from build123d import *

# Parameters (mm, degrees)
F1_DEPTH = 1


with BuildPart() as f1:
    # F0 (on Front) → F1 (new body)
    with BuildSketch(Plane.XZ):
        with BuildLine():
            Line((29.8694758117, 20.3505297415), (-28.1305241883, 20.3505297415))
            ThreePointArc((-28.1305241883, 20.3505297415), (-29.5447377507, 19.7647433039), (-30.1305241883, 18.3505297415))
            Line((-30.1305241883, 18.3505297415), (-30.1305241883, 10.3505297415))
            Line((-30.1305241883, 10.3505297415), (-29.0812929486, 3.7248891079))
            ThreePointArc((-29.0812929486, 3.7248891079), (-25.1305241883, 0.3505297415), (-21.179755428, 3.7248891079))
            Line((-21.179755428, 3.7248891079), (-20.1305241883, 10.3505297415))
            ThreePointArc((-20.1305241883, 10.3505297415), (-18.6660580942, 13.8860636474), (-15.1305241883, 15.3505297415))
            Line((-15.1305241883, 15.3505297415), (-13.2839401439, 15.3505297415))
            Line((-13.2839401439, 15.3505297415), (-4.2025822867, 15.3505297415))
            ThreePointArc((-4.2025822867, 15.3505297415), (-0.6670483807, 13.8860636474), (0.7974177133, 10.3505297415))
            ThreePointArc((0.7974177133, 10.3505297415), (2.2618838074, 6.8149958356), (5.7974177133, 5.3505297415))
            ThreePointArc((5.7974177133, 5.3505297415), (9.3329516193, 6.8149958356), (10.7974177133, 10.3505297415))
            ThreePointArc((10.7974177133, 10.3505297415), (12.2618838074, 13.8860636474), (15.7974177133, 15.3505297415))
            Line((15.7974177133, 15.3505297415), (27.8694758117, 15.3505297415))
            Line((27.8694758117, 15.3505297415), (61.8694758117, 15.3505297415))
            Line((61.8694758117, 15.3505297415), (73.9415339101, 15.3505297415))
            ThreePointArc((73.9415339101, 15.3505297415), (77.477067816, 13.8860636474), (78.9415339101, 10.3505297415))
            ThreePointArc((78.9415339101, 10.3505297415), (80.4060000042, 6.8149958356), (83.9415339101, 5.3505297415))
            ThreePointArc((83.9415339101, 5.3505297415), (87.477067816, 6.8149958356), (88.9415339101, 10.3505297415))
            ThreePointArc((88.9415339101, 10.3505297415), (90.4060000042, 13.8860636474), (93.9415339101, 15.3505297415))
            Line((93.9415339101, 15.3505297415), (103.0228917673, 15.3505297415))
            Line((103.0228917673, 15.3505297415), (104.8694758117, 15.3505297415))
            ThreePointArc((104.8694758117, 15.3505297415), (108.4050097177, 13.8860636474), (109.8694758117, 10.3505297415))
            Line((109.8694758117, 10.3505297415), (110.9187070514, 3.7248891079))
            ThreePointArc((110.9187070514, 3.7248891079), (114.8694758117, 0.3505297415), (118.820244572, 3.7248891079))
            Line((118.820244572, 3.7248891079), (119.8694758117, 10.3505297415))
            Line((119.8694758117, 10.3505297415), (119.8694758117, 18.3505297415))
            ThreePointArc((119.8694758117, 18.3505297415), (119.2836893741, 19.7647433039), (117.8694758117, 20.3505297415))
            Line((117.8694758117, 20.3505297415), (59.8694758117, 20.3505297415))
            Line((59.8694758117, 20.3505297415), (29.8694758117, 20.3505297415))
        make_face()
    extrude(amount=F1_DEPTH)


solid = f1.part
Build history of the part. All positions in model axes, mm. A direction names the side the tool comes from. Round coordinates to 2 decimals unless told otherwise and drop trailing zeros. Loops run counter-clockwise (first coordinate to the right, second up) from the corner with the lowest first, then second, coordinate; pieces in that order, holes last. Notation, with made-up numbers: (-15.75, 28.25) -> (-0.75, 28.25) arc R24 ccw to (-0.75, 54.25) -> close; hole circle Ø11 at (66.25, -38.75). An arc over 180 degrees is marked (long way). One line per item, written item: value. Start each with the question number.
Q1. Cut at C-C on x = 65.5. List the corners of the cut face in (y, z), plus the area to 3 significant figures.
Q2. Cut at B-B on y = -0.3. List the corners of the cut face in (x, z).
Q3. 3-axis set-ups, long thin cutter, end or side, ignore diameter. For faces 1 (the face through (108.37, -0.49, 13.92)), 2 (the face through (44, 0, 17)): which of +Z, -Z, +X, -X, +Y, -Y reach the whole face in a straight line?
Q4. Probe line 1 along X through (y, z) = (-0.2, 10.5); line 2 along X through (y, z) = (-0.45, 13.5); line 3 along Z through (x, y) = (37, -0.2). List the from-to ranges inside material, lowest first.
Q5. Cut at A-A on z = 12. List the corners of the cut face in (x, y).
Q6. Cut at D-D on x = 14. List the corners of the cut face in (y, z).
Q7. Drop a flat-ended pin along its axis: pin 1 Ø0.5 at (x, y) = (101, -0.5) entering from -Z. Give the stop position or say it passes through.
Computed:
1. outline: (-1, 15.35) -> (0, 15.35) -> (0, 20.35) -> (-1, 20.35) -> close
1. area: 5.00 mm²
2. outline: (-30.13, 10.35) -> (-29.08, 3.72) arc R4 ccw to (-21.18, 3.72) -> (-20.13, 10.35) arc R5 cw to (-15.13, 15.35) -> (-4.2, 15.35) arc R5 cw to (0.8, 10.35) arc R5 ccw to (10.8, 10.35) arc R5 cw to (15.8, 15.35) -> (73.94, 15.35) arc R5 cw to (78.94, 10.35) arc R5 ccw to (88.94, 10.35) arc R5 cw to (93.94, 15.35) -> (104.87, 15.35) arc R5 cw to (109.87, 10.35) -> (110.92, 3.72) arc R4 ccw to (118.82, 3.72) -> (119.87, 10.35) -> (119.87, 18.35) arc R2 ccw to (117.87, 20.35) -> (-28.13, 20.35) arc R2 ccw to (-30.13, 18.35) -> close
3. face 1: -Z, +Y, -Y
3. face 2: +Z, -Z, +X, -X, +Y
4. line 1: -30.13 to -20.13, 0.8 to 10.8, 78.94 to 88.94, 109.87 to 119.87
4. line 2: -30.13 to -19.01, -0.32 to 11.91, 77.82 to 90.06, 108.75 to 119.87
4. line 3: 15.35 to 20.35
5. outline: (-30.13, -1) -> (-19.85, -1) -> (-19.85, 0) -> (-30.13, 0) -> close; (0.52, -1) -> (11.08, -1) -> (11.08, 0) -> (0.52, 0) -> close; (78.66, -1) -> (89.22, -1) -> (89.22, 0) -> (78.66, 0) -> close; (109.59, -1) -> (119.87, -1) -> (119.87, 0) -> (109.59, 0) -> close
6. outline: (-1, 15.02) -> (0, 15.02) -> (0, 20.35) -> (-1, 20.35) -> close
7. pin 1: z = 15.35
